Input: dimensioned drawing with shaded views. Units: mm. Origin: part minimum x, y, z. A direction names the side the tool comes from. Give positions to 0.01 mm unless a question says otherwise; leave off trailing zeros. Write each loop counter-clockwise with the first axis right and the second up, starting at its lowest first coordinate (ties: lowest second). Pieces come first, ordered by that corner, then holes. Notation, with made-up numbers: (-17, 32) -> (-13, 32) arc R15 cw to (-13, 51) -> close; hole circle Ø8 at (82.5, -24). An arc over 180 degrees is marked (long way). Answer as a JSON object with one key per item and string values.
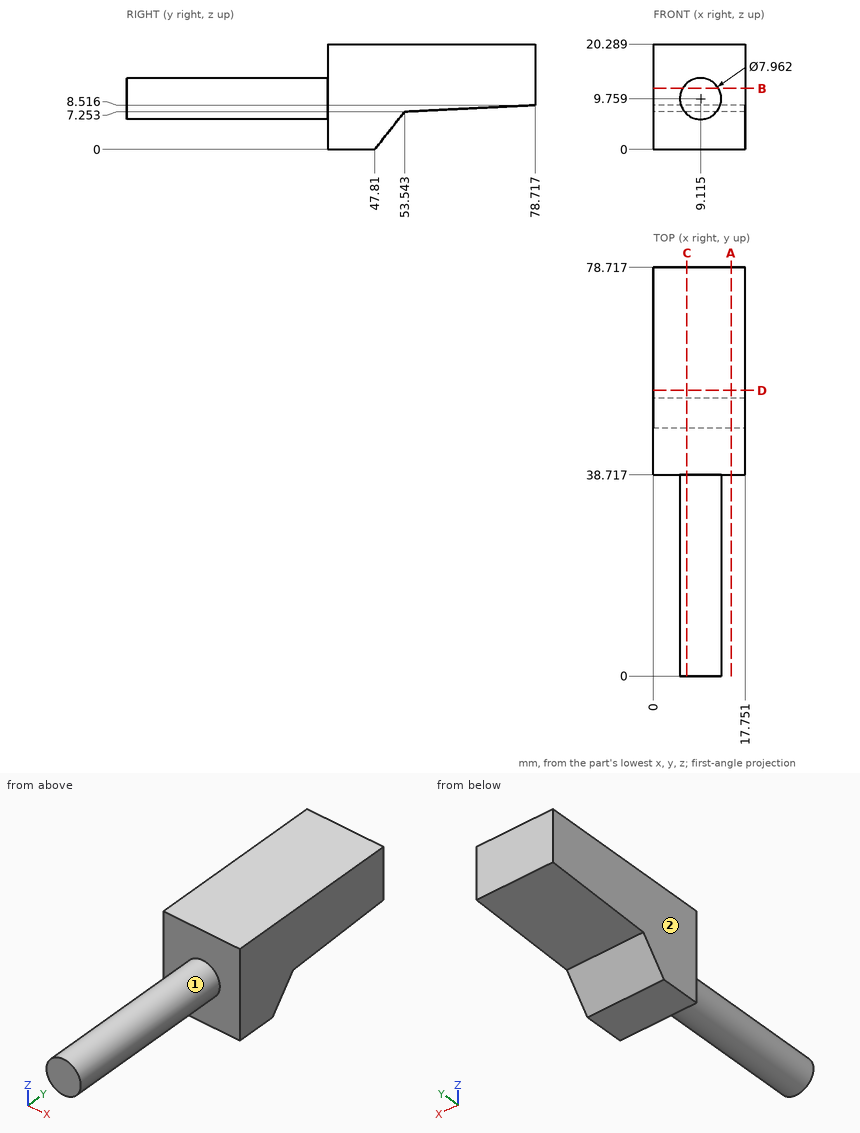
Q1. Cut plane D-D (y = 55). Return the cut outline in (x, z) (1 decimal).
Values:
{"outline": "(0, 7.3) -> (17.8, 7.3) -> (17.8, 20.3) -> (0, 20.3) -> close"}
Q2. Cut plane B-B (z = 11.75). Return the cut outline in (x, y), and give its area (3 significant figures).
Values:
{"outline": "(0, 38.72) -> (5.67, 38.72) -> (5.67, 0) -> (12.56, 0) -> (12.56, 38.72) -> (17.75, 38.72) -> (17.75, 78.72) -> (0, 78.72) -> close", "area": "977 mm²"}
Q3. Material intervals for L1, parallel to X at y = 6.5, z = 9.75 (1 decimal); L2, parallel to Y at x = 3.5, z = 9; L3, parallel to X at y = 33.5, z = 6.25 (1 decimal), sorted ascending. Write a range as from..to.
Values:
{"L1": "5.1..13.1", "L2": "38.72..78.72", "L3": "7.2..11"}
Q4. Cut plane A-A (x = 15). Return the cut outline in (y, z) (1 decimal), and give its area (3 significant figures).
Values:
{"outline": "(38.7, 0) -> (47.8, 0) -> (53.5, 7.3) -> (78.7, 8.5) -> (78.7, 20.3) -> (38.7, 20.3) -> close", "area": "592 mm²"}
Q5. Cut plane C-C (x = 6.5). Return the cut outline in (y, z) (1 decimal), and give its area (3 significant figures).
Values:
{"outline": "(0, 6.8) -> (38.7, 6.8) -> (38.7, 0) -> (47.8, 0) -> (53.5, 7.3) -> (78.7, 8.5) -> (78.7, 20.3) -> (38.7, 20.3) -> (38.7, 12.8) -> (0, 12.8) -> close", "area": "825 mm²"}
Q6. Set-up query: the marked faces 1 and 2. Return all of +Z, -Z, +X, -X, +Y, -Y with unobstructed straight access to the full face (end or side cutting, diameter ignored); none if empty.
Values:
{"face 1": "-Y", "face 2": "+Z, -Z, -X, +Y, -Y"}
Q7. First-contact query: P1, Ø5, axis at y = 10, z = 16.5, coming from the +X side; P2, Ø10, axis at x = 9, z = 5, coming from the -Y side; P3, Ø1, axis at x = 14, z = 7.5, coming from the -Y side; P4, Ø3, axis at x = 5.5, y = 25, coming from the -Z side. Flat tips, straight axial feed; report the tip coordinate or a pass-through.
Values:
{"P1": "through", "P2": "y = 0", "P3": "y = 38.72", "P4": "z = 6.39"}
